```python
from build123d import *

# Parameters (mm, degrees)
SM_BASE_FLANGE_1_DEPTH           = 125
SKETCH_3_W                       = 11
SKETCH_3_H                       = 19
CUT_EXTRUDE_1_DEPTH              = 1
SM_EDGE_FLANGE_1_STRIP_W         = 4.4
SM_EDGE_FLANGE_1_STRIP_H         = 1
SM_EDGE_FLANGE_1_STRIP_CUT_DEPTH = 15
SM_EDGE_FLANGE_1_DEPTH           = 15
SKETCH_7_R                       = 2.5
SKETCH_7_R_2                     = 2.2
CUT_EXTRUDE_2_DEPTH              = 1
SKETCH_8_R                       = 2.2
SKETCH_8_R_2                     = 2.5
CUT_EXTRUDE_3_DEPTH              = 1


# Sheet-metal steps are written as plain solids
with BuildPart() as part:
    # Sketch 1 → Базовая кромка1 (new, symmetric)
    with BuildSketch(Plane.XY):
        with BuildLine():
            Line((11, 14.7), (11, 16.5))
            ThreePointArc((11, 16.5), (10.648528137, 17.348528137), (9.8, 17.7))
            Line((9.8, 17.7), (1.2, 17.7))
            ThreePointArc((1.2, 17.7), (0.351471863, 17.348528137), (0, 16.5))
            Line((0, 16.5), (0, -16.5))
            ThreePointArc((0, -16.5), (0.351471863, -17.348528137), (1.2, -17.7))
            Line((1.2, -17.7), (9.8, -17.7))
            ThreePointArc((9.8, -17.7), (10.648528137, -17.348528137), (11, -16.5))
            Line((11, -16.5), (11, -14.7))
            Line((11, -14.7), (10, -14.7))
            Line((10, -14.7), (10, -16.5))
            ThreePointArc((10, -16.5), (9.941421356, -16.641421356), (9.8, -16.7))
            Line((9.8, -16.7), (1.2, -16.7))
            ThreePointArc((1.2, -16.7), (1.058578644, -16.641421356), (1, -16.5))
            Line((1, -16.5), (1, 16.5))
            ThreePointArc((1, 16.5), (1.058578644, 16.641421356), (1.2, 16.7))
            Line((1.2, 16.7), (9.8, 16.7))
            ThreePointArc((9.8, 16.7), (9.941421356, 16.641421356), (10, 16.5))
            Line((10, 16.5), (10, 14.7))
            Line((10, 14.7), (11, 14.7))
        make_face()
    extrude(amount=SM_BASE_FLANGE_1_DEPTH, both=True)

    # Эскиз3 → Вытянуть1 (cut)
    with BuildSketch(Plane(origin=(1, 0, 0), x_dir=(0, 0, -1), z_dir=(1, 0, 0))):
        with Locations((119.5, 0)):
            Rectangle(SKETCH_3_W, SKETCH_3_H)
    extrude(amount=-CUT_EXTRUDE_1_DEPTH, mode=Mode.SUBTRACT)

    # Ребро-кромка1 strip (across the edge) → Ребро-кромка1 strip cut (cut)
    with BuildSketch(Plane(origin=(1, -7.5, -114), x_dir=(0, 0, 1), z_dir=(0, 1, 0))):
        with Locations((-2, -0.5)):
            Rectangle(SM_EDGE_FLANGE_1_STRIP_W, SM_EDGE_FLANGE_1_STRIP_H)
    extrude(amount=SM_EDGE_FLANGE_1_STRIP_CUT_DEPTH, mode=Mode.SUBTRACT)

    # Ребро-кромка1 section (across the edge) → Ребро-кромка1 (add)
    with BuildSketch(Plane(origin=(1, -7.5, -114), x_dir=(0, 0, 1), z_dir=(0, 1, 0))):
        with BuildLine():
            Line((-1, 0.2), (-1, 8))
            Line((-1, 8), (0, 8))
            Line((0, 8), (0, 0.2))
            ThreePointArc((0, 0.2), (0.058578644, 0.058578644), (0.2, 0))
            Line((0.2, 0), (0.2, -1))
            ThreePointArc((0.2, -1), (-0.648528137, -0.648528137), (-1, 0.2))
        make_face()
    extrude(amount=SM_EDGE_FLANGE_1_DEPTH)

    # Эскиз7 → Вытянуть2 (cut)
    with BuildSketch(Plane(origin=(1, 0, 0), x_dir=(0, 0, -1), z_dir=(1, 0, 0))):
        with Locations(Location((65, 0, 0), (0, 0, 90))):
            Circle(SKETCH_7_R)
        with Locations(Location((50, 0, 0), (0, 0, 90))):
            Circle(SKETCH_7_R_2)
        with Locations(Location((1, 0, 0), (0, 0, 90))):
            Circle(SKETCH_7_R)
        with Locations(Location((-14, 0, 0), (0, 0, 90))):
            Circle(SKETCH_7_R_2)
    extrude(amount=-CUT_EXTRUDE_2_DEPTH, mode=Mode.SUBTRACT)

    # Эскиз8 → Вытянуть3 (cut)
    with BuildSketch(Plane(origin=(1, 0, 0), x_dir=(0, 0, -1), z_dir=(1, 0, 0))):
        with Locations(Location((-90, 0, 0), (0, 0, 90))):
            Circle(SKETCH_8_R)
        with Locations(Location((-75, 0, 0), (0, 0, 90))):
            Circle(SKETCH_8_R_2)
    extrude(amount=-CUT_EXTRUDE_3_DEPTH, mode=Mode.SUBTRACT)


solid = part.part
```
Verification items for the finished model (mm, model axes). A direction names the side the tool comes from. Give positions to 0.01 mm unless a question says otherwise; leave off trailing zeros. Loops run counter-clockwise (first coordinate to the right, second up) from the corner with the lowest first, then second, coordinate; pieces in that order, holes last.
1. Section check B-B, the plane x = 6. Enter the section's corners in (y, z), then the cut area to 3 significant figures.
2. Go/stop test with flat-tipped pins: pin 1 Ø5 at (x, y) = (6.5, -8.5) entering from +Z; pin 2 Ø5 at (y, z) = (0, 90) entering from +X; pin 3 Ø0.5 at (y, z) = (-3, -114.5) entering from +X. Record where each tip stops, or that it passes through.
3. Section check A-A, the plane z = 75. Enter the section's corners in (x, y).
4. Section check D-D, the plane z = -6. Enter the section's corners in (x, y).
5. Thickness scan on line 1 (Y direction, x = 9.25, z = -22); line 2 (X direction, y = 15.5, z = -92); line 3 (Z direction, x = 7.25, y = -7). Record the ranges inside material, lowest first.
6. Mould release check, pull along Y, two halves, no side actions. Record for faces 4 (the flat face through (4, 17, -125)), 5 (the cylindrical face through (0.51, -0.54, -3.44)), 6 (the flat face through (6, 17.7, 2)): released by +Y, released by -Y, zero draft, split by the parting line, or undercut.
7. Set-up check for faces 1 (the flat face through (5, 0, -115)), 2 (the flat face through (5, 16.7, 2)), 3 (the flat face through (5, 0, -114)): record each of +Z, -Z, +X, -X, +Y, -Y from which the full face is reachable in a straight line by a thin tool's end or side.
8. Section check C-C, the plane y = 0. Count the separate pieces of the cut face and the enclosed holes in it, then the cut area to 4 significant figures.
Geometry says:
1. outline: (-17.7, -125) - (-16.7, -125) - (-16.7, 125) - (-17.7, 125) - close; (-7.5, -115) - (7.5, -115) - (7.5, -114) - (-7.5, -114) - close; (16.7, -125) - (17.7, -125) - (17.7, 125) - (16.7, 125) - close
1. area: 515 mm2
2. pin 1: stops at z = -114
2. pin 2: stops at x = 1
2. pin 3: stops at x = 9
3. outline: (0, -16.5) arc R1.2 ccw to (1.2, -17.7) - (9.8, -17.7) arc R1.2 ccw to (11, -16.5) - (11, -14.7) - (10, -14.7) - (10, -16.5) arc R0.2 cw to (9.8, -16.7) - (1.2, -16.7) arc R0.2 cw to (1, -16.5) - (1, -2.5) - (0, -2.5) - close; (0, 2.5) - (1, 2.5) - (1, 16.5) arc R0.2 cw to (1.2, 16.7) - (9.8, 16.7) arc R0.2 cw to (10, 16.5) - (10, 14.7) - (11, 14.7) - (11, 16.5) arc R1.2 ccw to (9.8, 17.7) - (1.2, 17.7) arc R1.2 ccw to (0, 16.5) - close
4. outline: (0, -16.5) arc R1.2 ccw to (1.2, -17.7) - (9.8, -17.7) arc R1.2 ccw to (11, -16.5) - (11, -14.7) - (10, -14.7) - (10, -16.5) arc R0.2 cw to (9.8, -16.7) - (1.2, -16.7) arc R0.2 cw to (1, -16.5) - (1, 16.5) arc R0.2 cw to (1.2, 16.7) - (9.8, 16.7) arc R0.2 cw to (10, 16.5) - (10, 14.7) - (11, 14.7) - (11, 16.5) arc R1.2 ccw to (9.8, 17.7) - (1.2, 17.7) arc R1.2 ccw to (0, 16.5) - close
5. line 1: y = -17.7 to -16.7, 16.7 to 17.7
5. line 2: x = 0 to 1, 10 to 11
5. line 3: z = -115 to -114
6. face 4: zero draft
6. face 5: undercut
6. face 6: released by +Y
7. face 1: -Z, +X, -X
7. face 2: +Z, -Z
7. face 3: +Z, +X
8. separate pieces: 7
8. enclosed holes: 0
8. area: 219.5 mm2
